Read the model definition and answer for the solid it produces. Units are mm, in the model's axes. Face numbers are marked on the shaded views. A direction names the side the tool comes from. Give positions to 0.01 mm unless a question says otherwise; leave off trailing zeros. Order: outer loops, then holes, each group sorted by start corner. A loop starts at its lowest first (then second) coordinate and runs counter-clockwise, first axis right, second up. Notation, with made-up numbers: (21, 14) - (70, 14) arc R25 cw to (70, 44) - close; hole circle Ø6 at (-37.5, -22). An arc over 180 degrees is marked (long way). Write item = value, one per line.
```python
from build123d import *

# Parameters (mm, degrees)
SKETCH1_W                = 22
SKETCH1_H                = 65
BOSS_EXTRUDE1_DEPTH      = 18.6
FILLET1_R                = 4
BOSS_EXTRUDE2_DEPTH      = 9
BOSS_EXTRUDE2_DEPTH_BACK = 27.6
SKETCH2_R                = 2.65
CUT_EXTRUDE1_DEPTH       = 8
CUT_EXTRUDE2_DEPTH       = 8
SKETCH5_R                = 1.25
CUT_EXTRUDE3_DEPTH       = 51.16781837
BOSS_EXTRUDE3_START      = -7
SKETCH6_W                = 5
SKETCH6_H                = 10
SKETCH6_R                = 1.5
BOSS_EXTRUDE3_DEPTH      = 3
SKETCH7_R                = 2.85
SKETCH7_R_2              = 2.65
BOSS_EXTRUDE4_DEPTH      = 0.5
SKETCH8_R                = 2
BOSS_EXTRUDE5_DEPTH      = 2
SKETCH9_R                = 1.5
CUT_EXTRUDE4_DEPTH       = 48.843599363
SKETCH10_W               = 27.728887241
SKETCH10_H               = 31.632468454
CUT_EXTRUDE5_DEPTH       = 1
SKETCH11_R               = 16.996731029
SKETCH11_R_2             = 11
CUT_EXTRUDE6_DEPTH       = 28
CUT_EXTRUDE7_DEPTH       = 16.8
FILLET2_R                = 3


with BuildPart() as part:
    # Sketch1 → Boss-Extrude1 (new body)
    with BuildSketch(Plane.XY):
        Rectangle(SKETCH1_W, SKETCH1_H)
    extrude(amount=BOSS_EXTRUDE1_DEPTH)

    # Fillet1
    fillet1_edges = [part.edges().sort_by_distance(p)[0] for p in [
        (-11, 32.5, 9.3),
        (11, 32.5, 9.3),
    ]]
    fillet(fillet1_edges, radius=FILLET1_R)

    # Sketch2 → Boss-Extrude2 (add, two sides: drawn at the far end of the back side and taken through both)
    with BuildSketch(Plane.XY.offset(18.6).offset(-BOSS_EXTRUDE2_DEPTH_BACK)):
        with Locations((0, 21.5)):
            Circle(SKETCH2_R)
    extrude(amount=BOSS_EXTRUDE2_DEPTH + BOSS_EXTRUDE2_DEPTH_BACK)

    # Sketch3 → Cut-Extrude1 (cut)
    with BuildSketch(Plane.XY.offset(27.6)):
        with BuildLine():
            Line((-1.989974874, 23.25), (1.989974874, 23.25))
            ThreePointArc((1.989974874, 23.25), (0, 24.15), (-1.989974874, 23.25))
        make_face()
        with BuildLine():
            Line((-1.989974874, 19.75), (1.989974874, 19.75))
            ThreePointArc((1.989974874, 19.75), (0, 18.85), (-1.989974874, 19.75))
        make_face()
    extrude(amount=-CUT_EXTRUDE1_DEPTH, mode=Mode.SUBTRACT)

    # Sketch4 → Cut-Extrude2 (cut)
    with BuildSketch(Plane(origin=(0, 0, -9), x_dir=(-1, 0, 0), z_dir=(0, 0, -1))):
        with BuildLine():
            Line((-1.989974874, 19.75), (1.989974874, 19.75))
            ThreePointArc((1.989974874, 19.75), (0, 18.85), (-1.989974874, 19.75))
        make_face()
        with BuildLine():
            Line((1.989974874, 23.25), (-1.989974874, 23.25))
            ThreePointArc((-1.989974874, 23.25), (0, 24.15), (1.989974874, 23.25))
        make_face()
    extrude(amount=-CUT_EXTRUDE2_DEPTH, mode=Mode.SUBTRACT)

    # Sketch5 → Cut-Extrude3 (cut, through all)
    with BuildSketch(Plane(origin=(0, 0, -9), x_dir=(-1, 0, 0), z_dir=(0, 0, -1))):
        with Locations((0, 21.5)):
            Circle(SKETCH5_R)
    extrude(amount=-CUT_EXTRUDE3_DEPTH, mode=Mode.SUBTRACT)

    # Sketch6 → Boss-Extrude3 (add)
    with BuildSketch(Plane.XY.offset(18.6).offset(BOSS_EXTRUDE3_START)):
        with Locations((0, 32.5)):
            Rectangle(SKETCH6_W, SKETCH6_H)
        with Locations((0, 35)):
            Circle(SKETCH6_R, mode=Mode.SUBTRACT)
    extrude(amount=-BOSS_EXTRUDE3_DEPTH)

    # Sketch7 → Boss-Extrude4 (add)
    with BuildSketch(Plane(origin=(0, 0, 0), x_dir=(-1, 0, 0), z_dir=(0, 0, -1))):
        with Locations(Location((0, 21.5, 0), (0, 0, 180))):
            Circle(SKETCH7_R)
        with Locations(Location((0, 21.5, 0), (0, 0, 221.328658646))):
            Circle(SKETCH7_R_2, mode=Mode.SUBTRACT)
    extrude(amount=BOSS_EXTRUDE4_DEPTH)

    # Sketch8 → Boss-Extrude5 (add)
    with BuildSketch(Plane(origin=(0, 0, 0), x_dir=(-1, 0, 0), z_dir=(0, 0, -1))):
        with Locations(Location((0, 10.5, 0), (0, 0, 180))):
            Circle(SKETCH8_R)
    extrude(amount=BOSS_EXTRUDE5_DEPTH)

    # Sketch9 → Cut-Extrude4 (cut, through all)
    with BuildSketch(Plane(origin=(0, 0, 0), x_dir=(-1, 0, 0), z_dir=(0, 0, -1))):
        with Locations((-8.5, 0.5)):
            Circle(SKETCH9_R)
        with Locations(Location((8.5, 0.5, 0), (0, 0, 180))):
            Circle(SKETCH9_R)
    extrude(amount=-CUT_EXTRUDE4_DEPTH, mode=Mode.SUBTRACT)

    # Sketch10 → Cut-Extrude5 (cut)
    with BuildSketch(Plane(origin=(0, 0, 0), x_dir=(-1, 0, 0), z_dir=(0, 0, -1))):
        with Locations((0.201909374, -20.316234227)):
            Rectangle(SKETCH10_W, SKETCH10_H)
    extrude(amount=-CUT_EXTRUDE5_DEPTH, mode=Mode.SUBTRACT)

    # Sketch11 → Cut-Extrude6 (cut)
    with BuildSketch(Plane.XZ.offset(32.5)):
        with Locations((0, 9.8)):
            Circle(SKETCH11_R)
        with Locations((0, 9.8)):
            Circle(SKETCH11_R_2, mode=Mode.SUBTRACT)
    extrude(amount=-CUT_EXTRUDE6_DEPTH, mode=Mode.SUBTRACT)

    # Sketch12 → Cut-Extrude7 (cut)
    with BuildSketch(Plane.XZ.offset(32.5)):
        with BuildLine():
            Line((6.6, 18.6), (-6.6, 18.6))
            ThreePointArc((-6.6, 18.6), (-11, 9.8), (-6.6, 1))
            Line((-6.6, 1), (6.6, 1))
            ThreePointArc((6.6, 1), (11, 9.8), (6.6, 18.6))
        make_face()
        with BuildLine():
            Line((6.187083319, 17.4), (-6.187083319, 17.4))
            ThreePointArc((-6.187083319, 17.4), (-9.8, 9.8), (-6.187083319, 2.2))
            Line((-6.187083319, 2.2), (6.187083319, 2.2))
            ThreePointArc((6.187083319, 2.2), (9.8, 9.8), (6.187083319, 17.4))
        make_face(mode=Mode.SUBTRACT)
    extrude(amount=-CUT_EXTRUDE7_DEPTH, mode=Mode.SUBTRACT)

    # Fillet2
    # the kernel refuses this fillet: 3 mm, written as the material it takes off along each edge
    with BuildSketch(Plane(origin=(0, -32.5, 9.8), x_dir=(-0.08233193306434959, 0, -0.9966049632617165), z_dir=(-0.9966049632617165, 0, 0.08233193306434959))) as fillet2_piece_1:
        with BuildLine():
            CenterArc((9.8 - FILLET2_R, -FILLET2_R), FILLET2_R, 0, 90)
            Line((9.8 - FILLET2_R, 0), (9.8, 0))
            Line((9.8, 0), (9.8, -FILLET2_R))
        make_face()
    revolve(axis=Axis((0, -32.5, 9.8), (0, -1, 0)), revolution_arc=189.445235963, mode=Mode.SUBTRACT)
    with BuildSketch(Plane(origin=(0, -32.5, 9.8), x_dir=(0.08233193306435141, 0, 0.9966049632617163), z_dir=(0.9966049632617163, 0, -0.08233193306435141))) as fillet2_piece_2:
        with BuildLine():
            CenterArc((9.8 - FILLET2_R, -FILLET2_R), FILLET2_R, 0, 90)
            Line((9.8 - FILLET2_R, 0), (9.8, 0))
            Line((9.8, 0), (9.8, -FILLET2_R))
        make_face()
    revolve(axis=Axis((0, -32.5, 9.8), (0, -1, 0)), revolution_arc=189.445235963, mode=Mode.SUBTRACT)


solid = part.part
```
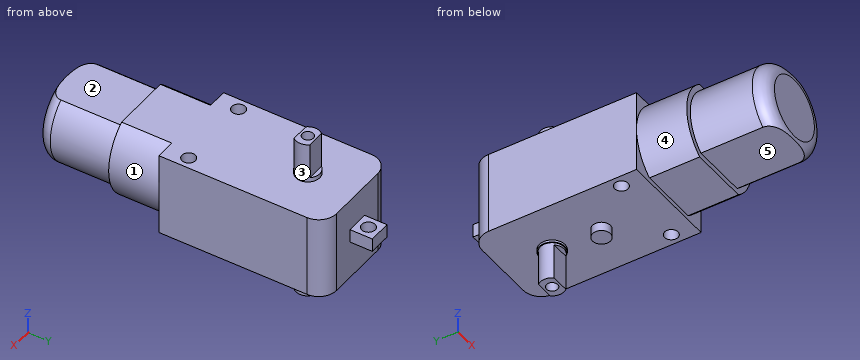
1. Section C-C (y = -24.5) is taken. Determine the outline of the cut face in (x, z).
Recorded:
outline = (-6.19, 2.2) - (6.19, 2.2) arc R9.8 ccw to (6.19, 17.4) - (-6.19, 17.4) arc R9.8 ccw to start
2. Straight lines are drawn through the part: L1, parallel to Y at x = 0, z = 10.9; L2, parallel to Y at x = 0, z = 20.5; L3, parallel to X at y = 0, z = 6. For each, find the intervals that lie inside material, in ascending order. Write a range as [from, to].
Recorded:
L1 = [-32.5, 20.25], [22.75, 33.5], [36.5, 37.5]
L2 = [19.75, 20.25], [22.75, 23.25]
L3 = [-11, -9.91], [-7.09, 7.09], [9.91, 11]
3. For the marked faces 1, 2, 3, 4 and 5, determine the directions among +Z, -Z, +X, -X, +Y, -Y from which every point of the face is accessible in a straight line to the end or side of a thin tool.
Recorded:
face_1 = +X, -Y
face_2 = +Z, +X, -X, -Y
face_3 = +Z
face_4 = -X, -Y
face_5 = -Z, +X, -X, -Y
4. Section A-A (z = 23.5) is taken. Determine the outline of the cut face in (x, y).
Recorded:
outline = (-1.99, 19.75) - (1.99, 19.75) arc R2.65 ccw to (1.99, 23.25) - (-1.99, 23.25) arc R2.65 ccw to start; hole circle Ø2.5 at (0, 21.5)
5. Section B-B (y = 15.5) is taken. Determine the outline of the cut face in (x, z).
Recorded:
outline = (-11, 0) - (11, 0) - (11, 18.6) - (-11, 18.6) - close
6. Flat-ended cylindrical pins translate along their axes: pin 1 (2.5 mm diameter, centred on x = -0.5, y = 34.5, fed in from -Z); pin 2 (5.5 mm diameter, centred on x = -3, y = -10.5, fed in from -Z); pin 3 (2 mm diameter, centred on x = 8.5, z = 12.5, fed in from -Y); pin 4 (3 mm diameter, centred on y = -8.5, z = 22, fed in from +X). Find the tip coordinate at first contact, or state that the pin passes through.
Recorded:
pin_1 = 8.6
pin_2 = 1
pin_3 = -32.28
pin_4 = through
